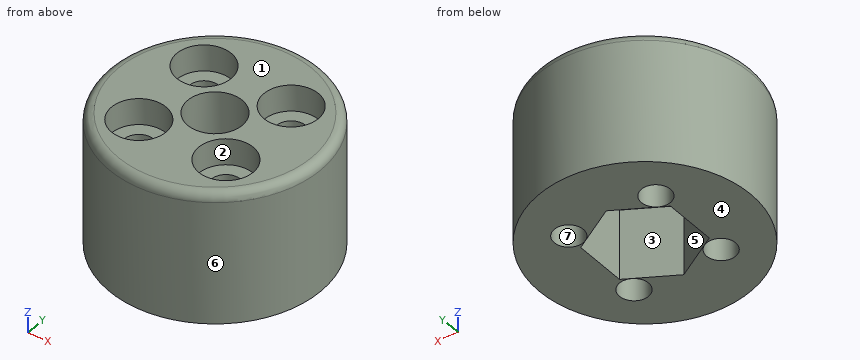
```python
from build123d import *

# Parameters (mm, degrees)
SKETCH_R        = 12
PAD_DEPTH       = 15
SKETCH001_R     = 1.65
POCKET_DEPTH    = 15.001
POCKET001_DEPTH = 8
SKETCH003_R     = 3.1
POCKET002_DEPTH = 7.001
SKETCH004_R     = 3.1
PAD001_DEPTH    = 0.2
SKETCH005_R     = 3.1
POCKET003_DEPTH = 3
FILLET_R        = 1
SKETCH006_R     = 1.65
PAD002_DEPTH    = 0.2


with BuildPart() as part:
    # Sketch → Pad (new body)
    with BuildSketch(Plane.XY):
        Circle(SKETCH_R)
    extrude(amount=PAD_DEPTH)

    # Sketch001 (on Face2 of Pad) → Pocket (cut, through all)
    with BuildSketch(Plane(origin=(0, 0, 0), x_dir=(1, 0, 0), z_dir=(0, 0, -1))):
        with Locations((-4.949747, 4.949747)):
            Circle(SKETCH001_R)
        with Locations((4.949747, 4.949747)):
            Circle(SKETCH001_R)
        with Locations((4.949747, -4.949747)):
            Circle(SKETCH001_R)
        with Locations((-4.949747, -4.949747)):
            Circle(SKETCH001_R)
    extrude(amount=-POCKET_DEPTH, mode=Mode.SUBTRACT)

    # Sketch002 (on Face2 of Pocket) → Pocket001 (cut)
    with BuildSketch(Plane(origin=(0, 0, 0), x_dir=(1, 0, 0), z_dir=(0, 0, -1))):
        Polygon((5.1, 2.944486), (0, 5.888973), (-5.1, 2.944486), (-5.1, -2.944486), (0, -5.888973), (5.1, -2.944486), align=None)
    extrude(amount=-POCKET001_DEPTH, mode=Mode.SUBTRACT)

    # Sketch003 (on Face14 of Pocket001) → Pocket002 (cut, through all)
    with BuildSketch(Plane(origin=(0, 0, 8), x_dir=(1, 0, 0), z_dir=(0, 0, -1))):
        Circle(SKETCH003_R)
    extrude(amount=-POCKET002_DEPTH, mode=Mode.SUBTRACT)

    # Sketch004 (on Face15 of Pocket002) → Pad001 (join)
    with BuildSketch(Plane(origin=(0, 0, 8), x_dir=(1, 0, 0), z_dir=(0, 0, -1))):
        Circle(SKETCH004_R)
    extrude(amount=-PAD001_DEPTH)

    # Sketch005 (on Face3 of Pad001) → Pocket003 (cut)
    with BuildSketch(Plane.XY.offset(15)):
        with Locations((4.949747, 4.949747)):
            Circle(SKETCH005_R)
        with Locations((4.949747, -4.949747)):
            Circle(SKETCH005_R)
        with Locations((-4.949747, -4.949747)):
            Circle(SKETCH005_R)
        with Locations((-4.949747, 4.949747)):
            Circle(SKETCH005_R)
    extrude(amount=-POCKET003_DEPTH, mode=Mode.SUBTRACT)

    # Fillet
    fillet_edges = [part.edges().sort_by_distance(p)[0] for p in [
        (-12, 0, 15),
    ]]
    fillet(fillet_edges, radius=FILLET_R)

    # Sketch006 (on Face22 of Fillet) → Pad002 (join)
    with BuildSketch(Plane(origin=(0, 0, 8), x_dir=(1, 0, 0), z_dir=(0, 0, -1))):
        with Locations((-4.949747, 4.949747)):
            Circle(SKETCH006_R)
        with Locations((4.949747, 4.949747)):
            Circle(SKETCH006_R)
        with Locations((4.949747, -4.949747)):
            Circle(SKETCH006_R)
        with Locations((-4.949747, -4.949747)):
            Circle(SKETCH006_R)
    extrude(amount=-PAD002_DEPTH)


solid = part.part
```
Design review of the part built by this model. Coordinates are the model's own, in mm. Face numbers are marked on the shaded views. A direction names the side the tool comes from. Coordinates: 2 decimals unless noted, no trailing zeros. Write each loop counter-clockwise with the first axis right and the second up, starting at its lowest first coordinate (ties: lowest second). Pieces come first, ordered by that corner, then holes.
1) Mouldability with a two-part tool opening along Y and no side actions: class the marked faces 4, 5, 6 and 7 as +Y half, -Y half, draft (parallel to the pull), parting line (faces both ways), or undercut.
2) Add section B-B (z = 11). Write out the cut boundary in (x, y).
3) Add section A-A (y = 0). Write out the cut boundary in (x, z).
4) Add section D-D (z = 7). Write out the cut boundary in (x, y).
5) Machinability: for the marked faces 1, 2 and 3, which of the approach directions +Z, -Z, +X, -X, +Y, -Y give a long, thin tool a straight path to every point of the face, cutting with its end or side? Answer none if there is none.
6) Insertion check: pin 1 (1.6 mm diameter, centred on x = 4.5, y = -5, fed in from -Z); pin 2 (5 mm diameter, centred on x = 4.5, z = 2.5, fed in from -Y); pin 3 (1 mm diameter, centred on y = -9, z = 2.5, fed in from +X). Each pin has a flat end and moves straight along its axis. Give the tip position at first contact, or say it passes through.
7) Add section C-C (z = 13.5). Write out the cut boundary in (x, y).
8) To check wall thickness, follow L1, parallel to X at y = 4, z = 10; L2, parallel to Y at x = 5.5, z = 4; L3, parallel to Y at x = -2.5, z = 14. State the ranges of each line that lie inside material, in increasing order.
Check result:
1. face 4: draft
1. face 5: undercut
1. face 6: parting line
1. face 7: undercut
2. outline: circle Ø24 at (0, 0); hole circle Ø3.3 at (-4.95, -4.95); hole circle Ø3.3 at (-4.95, 4.95); hole circle Ø6.2 at (0, 0); hole circle Ø3.3 at (4.95, -4.95); hole circle Ø3.3 at (4.95, 4.95)
3. outline: (-12, 0) - (-5.1, 0) - (-5.1, 8) - (5.1, 8) - (5.1, 0) - (12, 0) - (12, 14) arc R1 ccw to (11, 15) - (3.1, 15) - (3.1, 8.2) - (-3.1, 8.2) - (-3.1, 15) - (-11, 15) arc R1 ccw to (-12, 14) - close
4. outline: circle Ø24 at (0, 0); hole circle Ø3.3 at (-4.95, -4.95); hole circle Ø3.3 at (-4.95, 4.95); hole (-5.1, -2.94) - (0, -5.89) - (5.1, -2.94) - (5.1, 2.94) - (0, 5.89) - (-5.1, 2.94) - close; hole circle Ø3.3 at (4.95, -4.95); hole circle Ø3.3 at (4.95, 4.95)
5. face 1: +Z, +X, -X, +Y, -Y
5. face 2: +Z
5. face 3: -Z
6. pin 1: stops at z = 8
6. pin 2: stops at y = -11.83
6. pin 3: stops at x = 8.47
7. outline: circle Ø24 at (0, 0); hole circle Ø6.2 at (-4.95, -4.95); hole circle Ø6.2 at (-4.95, 4.95); hole circle Ø6.2 at (0, 0); hole circle Ø6.2 at (4.95, -4.95); hole circle Ø6.2 at (4.95, 4.95)
8. L1: x = -11.31 to -6.3, -3.6 to 3.6, 6.3 to 11.31
8. L2: y = -10.67 to -6.51, -3.39 to 3.39, 6.51 to 10.67
8. L3: y = -11.74 to -6.85, -3.05 to -1.83, 1.83 to 3.05, 6.85 to 11.74
